from build123d import *

# Parameters (mm, degrees)
SKETCH1_W           = 25
SKETCH1_H           = 7.15
BOSS_EXTRUDE1_DEPTH = 12
BOSS_EXTRUDE2_DEPTH = 3
CUT_EXTRUDE1_DEPTH  = 21
SKETCH4_R           = 8.65
CUT_EXTRUDE2_DEPTH  = 10
CHAMFER1_SIZE       = 5
CHAMFER1_SIZE2      = 20
CHAMFER2_SIZE       = 5
SKETCH6_R           = 1.05
CUT_EXTRUDE3_DEPTH  = 10
CUT_EXTRUDE4_DEPTH  = 4.5
FILLET1_R           = 3
FILLET2_R           = 1.5


with BuildPart() as part:
    # Sketch1 → Boss-Extrude1 (new body)
    with BuildSketch(Plane.XY):
        with Locations((12.5, 3.575)):
            Rectangle(SKETCH1_W, SKETCH1_H)
    extrude(amount=BOSS_EXTRUDE1_DEPTH)

    # Sketch2 → Boss-Extrude2 (add)
    with BuildSketch(Plane(origin=(0, 7.15, 0), x_dir=(1, 0, 0), z_dir=(0, 1, 0))):
        with BuildLine():
            Line((15, -12), (15, -6))
            Line((15, -6), (15, 0))
            Line((15, 0), (-5.804949202, 4.737516245))
            ThreePointArc((-5.804949202, 4.737516245), (-19.262380692, -6), (-5.804949202, -16.737516245))
            Line((-5.804949202, -16.737516245), (15, -12))
        make_face()
    extrude(amount=-BOSS_EXTRUDE2_DEPTH)

    # Sketch3 → Cut-Extrude1 (cut)
    with BuildSketch(Plane.XZ.offset(-4.15)):
        Polygon((2.25, 6), (2.25, 12), (0, 12), (0, 0), (2.25, 0), align=None)
    extrude(amount=CUT_EXTRUDE1_DEPTH, mode=Mode.SUBTRACT)

    # Sketch4 → Cut-Extrude2 (cut)
    with BuildSketch(Plane.XZ.offset(-4.15)):
        with Locations((-8.25, 6)):
            Circle(SKETCH4_R)
    extrude(amount=-CUT_EXTRUDE2_DEPTH, mode=Mode.SUBTRACT)

    # Chamfer1
    chamfer1_edges = [part.edges().sort_by_distance(p)[0] for p in [
        (25, 7.15, 6),
    ]]
    chamfer1_side = [part.faces().sort_by_distance(p)[0] for p in [
        (25, 3.575, 6),
    ]]
    chamfer(chamfer1_edges, length=CHAMFER1_SIZE, length2=CHAMFER1_SIZE2, reference=chamfer1_side[0])

    # Chamfer2
    chamfer2_edges = [part.edges().sort_by_distance(p)[0] for p in [
        (25, 1.075, 0),
        (25, 1.075, 12),
    ]]
    chamfer(chamfer2_edges, length=CHAMFER2_SIZE)

    # Sketch6 → Cut-Extrude3 (cut)
    with BuildSketch(Plane(origin=(0, 7.15, 0), x_dir=(1, 0, 0), z_dir=(0, 1, 0))):
        with Locations((7.829893366, -6)):
            Circle(SKETCH6_R)
        with Locations((17.829893366, -6)):
            Circle(SKETCH6_R)
    extrude(amount=-CUT_EXTRUDE3_DEPTH, mode=Mode.SUBTRACT)

    # Sketch7 → Cut-Extrude4 (cut)
    with BuildSketch(Plane(origin=(0, 7.15, 0), x_dir=(1, 0, 0), z_dir=(0, 1, 0))):
        with BuildLine():
            Line((7.829893366, -2), (17.829893366, -2))
            ThreePointArc((17.829893366, -2), (21.829893366, -6), (17.829893366, -10))
            Line((17.829893366, -10), (7.829893366, -10))
            ThreePointArc((7.829893366, -10), (3.829893366, -6), (7.829893366, -2))
        make_face()
    extrude(amount=-CUT_EXTRUDE4_DEPTH, mode=Mode.SUBTRACT)

    # Fillet1
    fillet1_edges = [part.edges().sort_by_distance(p)[0] for p in [
        (2.25, 2.075, 0),
        (2.25, 2.075, 12),
    ]]
    fillet(fillet1_edges, radius=FILLET1_R)

    # Fillet2
    fillet2_edges = [part.edges().sort_by_distance(p)[0] for p in [
        (2.25, 4.15, 6),
        (10.125, 4.15, 12),
        (3.128679656, 4.15, 11.121320344),
        (3.128679656, 4.15, 0.878679656),
        (10.125, 4.15, 0),
    ]]
    fillet(fillet2_edges, radius=FILLET2_R)


solid = part.part
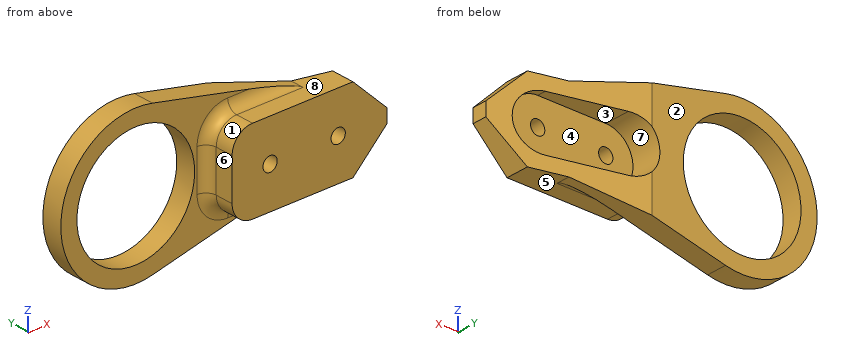
Model file for the job. Use its own axes, mm. Face numbers are marked on the shaded views. A direction names the side the tool comes from. Coordinates: 2 decimals unless noted, no trailing zeros. Order: outer loops, then holes, each group sorted by start corner. A loop starts at its lowest first (then second) coordinate and runs counter-clockwise, first axis right, second up. Notation, with made-up numbers: M 86.25,70 L 125.25,70 A24 ccw 125.25,83 Z; hole C 10,25.25 d7. An arc over 180 degrees is marked long. Return JSON: item names as keys, results as strings.
1. Saw through at D-D (y = 0.5). Give the cut face in (x, z), and give its area (3 significant figures).
Ans:
{"outline": "M 2.25,3 A3 ccw 5.25,0 L 20,0 L 25,5 L 25,7 L 20,12 L 5.25,12 A3 ccw 2.25,9 Z; hole C 7.83,6 d2.1; hole C 17.83,6 d2.1", "area": "237 mm^2"}
2. Saw through at C-C (y = 5.75). Give the cut face in (x, z).
Ans:
{"outline": "M -5.8,-4.74 L 10.6,-1 L 10.6,2 L 7.83,2 A4 cw 7.83,10 L 10.6,10 L 10.6,13 L -5.8,16.74 A11.01 ccw long Z; hole C -8.25,6 d17.3"}
3. Pull direction X, two halves, no side cores. Call the marked faces 1, 2, 3 and 4: +X half, -X half, draft (parallel to the pull), parting line (faces both ways), or undercut.
Ans:
{"face 1": "-X half", "face 2": "draft", "face 3": "undercut", "face 4": "undercut"}
4. Tool access for the marked faces 5, 6, 7 and 8: list every direction of +Z, -Z, +X, -X, +Y, -Y with a clear straight run to the whole face (end or side of a thin tool).
Ans:
{"face 5": "-Z, +X, -Y", "face 6": "+Z, -Z, -X, -Y", "face 7": "+Y", "face 8": "+Z, +X, -Y"}
5. Saw through at B-B (z = 6). Give the cut face in (x, y), and give its area (3 significant figures).
Ans:
{"outline": "M -19.26,4.15 L -16.9,4.15 L -16.9,7.15 L -19.26,7.15 Z; M 0.4,4.15 L 0.75,4.15 A1.5 cw 2.25,2.65 L 2.25,0 L 6.78,0 L 6.78,2.65 L 3.83,2.65 L 3.83,7.15 L 0.4,7.15 Z; M 8.88,0 L 16.78,0 L 16.78,2.65 L 8.88,2.65 Z; M 18.88,0 L 25,0 L 25,2.15 L 21.83,2.94 L 21.83,2.65 L 18.88,2.65 Z", "area": "69.1 mm^2"}
6. Saw through at A-A (x = -8.25). Give the cut face in (y, z).
Ans:
{"outline": "M 4.15,-5.01 L 7.15,-5.01 L 7.15,-2.65 L 4.15,-2.65 Z; M 4.15,14.65 L 7.15,14.65 L 7.15,17.01 L 4.15,17.01 Z"}
7. Drill centre lines: probe 1 along X at (y, z) = (0.55, 6); probe 2 along Z at (x, y) = (15, 4); probe 3 along X at (y, z) = (1, 5.5). Where is each one in solid material? Low to high.
Ans:
{"probe 1": "2.25 to 6.78, 8.88 to 16.78, 18.88 to 25", "probe 2": "0 to 2, 10 to 12", "probe 3": "2.25 to 6.91, 8.75 to 16.91, 18.75 to 25"}
8. Flat gauge pins, fed straight in: pin 1 (1.7 mm diameter, centred on x = 17.83, z = 6, fed in from +Y); pin 2 (9 mm diameter, centred on x = 9.5, z = 7, fed in from +Y); pin 3 (3 mm diameter, centred on x = -6, y = 4.5, fed in from +Z); pin 4 (6 mm diameter, centred on x = 9.5, z = 9, fed in from +Y). Where does each tip first touch, or does it go through?
Ans:
{"pin 1": "through", "pin 2": "y = 6.98", "pin 3": "z = 16.99", "pin 4": "y = 6.75"}
